Part model, mm, in its own coordinate system. A direction names the side the tool comes from. Coordinates: 2 decimals unless noted, no trailing zeros. Loops run counter-clockwise (first coordinate to the right, second up) from the corner with the lowest first, then second, coordinate; pieces in that order, holes last. Notation, with made-up numbers: (39.5, 80) -> (85.5, 80) arc R15 cw to (85.5, 98) -> close; hole circle Ø9 at (-0.75, -1.5). An arc over 180 degrees is marked (long way). One line per question, with ' | ' between items. Start each with the question number.
1) Cut at C-C (z = 51.5). List the corners of the cut face in (x, y), plus the area to 3 significant figures.
2) Cut at D-D (y = 26). Count the separate pieces of the cut face and the enclosed holes in it, plus the area to 3 significant figures.
3) Cut at A-A (x = 0). List the corners of the cut face in (y, z), plus the area to 4 significant figures.
4) Two-plate mould, pull along X, no slides. Class faces 1 (the face through (36.46, 0.8, 26.82)), 2 (the face through (31.457, -0.798, 58.2)), 3 (the face through (-65.41, 0.8, 3.84)), 4 (the face through (-1, 57, 99)): released by +X, released by -X, zero draft, split by the parting line, or undercut.
5) Drop flat-ended pins along their axis: pin 1 (4 mm diameter, centred on y = 22.5, z = 204, fed in from -X); pin 2 (11 mm diameter, centred on x = 65.5, y = 16.5, fed in from -Z); pin 3 (1 mm diameter, centred on y = -28.5, z = 88.5, fed in from +X). Give the stop position or say it passes through.
6) 3-axis set-ups, long thin cutter, end or side, ignore diameter. For faces 5 (the face through (-69, -1, 90)), 6 (the face through (-2.539, 19.334, 102.675)), 7 (the face through (31.86, 0.8, 223.22)), 8 (the face through (68, -1, 90)): which of +Z, -Z, +X, -X, +Y, -Y reach the whole face in a straight line?
7) Probe L1, parallel to Z at x = -17, y = -52; L2, parallel to Y at x = 0, z = 102; L3, parallel to Z at x = -6.5, y = -8. List the from-to ranges inside material, lowest first. Write a range as from..to.
from build123d import *

# Parameters (mm, degrees)
F1_DEPTH  = 57
F2_R      = 18
F3_R      = 10
F5_DEPTH  = 114
F6_R      = 5
F8_DEPTH  = 114
F9_R      = 10
F10_R     = 19.5
F11_DEPTH = 25


with BuildPart() as f1:
    # F0 (on Front) → F1 (new body, symmetric)
    with BuildSketch(Plane.XZ):
        Polygon((-70, 0), (70, 0), (50, 90), (112.991273, 90), (50, 250), (-50, 250), (-112.991273, 90), (-50, 90), align=None)
    extrude(amount=F1_DEPTH, both=True)

    # F2
    f2_edges = [f1.edges().sort_by_distance(p)[0] for p in [
        (50, 0, 250),
        (-50, 0, 250),
        (112.991273, 0, 90),
        (-112.991273, 0, 90),
    ]]
    fillet(f2_edges, radius=F2_R)

    # F3
    f3_edges = [f1.edges().sort_by_distance(p)[0] for p in [
        (70, 0, 0),
        (-70, 0, 0),
    ]]
    fillet(f3_edges, radius=F3_R)

    # F4 (on face) → F5 (cut, through all)
    with BuildSketch(Plane.XZ.offset(57)):
        Polygon((-38.834599, 25), (38.834599, 25), (24.390154, 90), (-24.390154, 90), align=None)
    extrude(amount=-F5_DEPTH, mode=Mode.SUBTRACT)

    # F6
    f6_edges = [f1.edges().sort_by_distance(p)[0] for p in [
        (-38.834599, 0, 25),
        (38.834599, 0, 25),
        (-24.390154, 0, 90),
        (24.390154, 0, 90),
    ]]
    fillet(f6_edges, radius=F6_R)

    # F7 (on face) → F8 (cut, through all)
    with BuildSketch(Plane.XZ.offset(57)):
        Polygon((-76.281201, 115), (76.281201, 115), (32.9747, 225), (-32.9747, 225), align=None)
    extrude(amount=-F8_DEPTH, mode=Mode.SUBTRACT)

    # F9
    f9_edges = [f1.edges().sort_by_distance(p)[0] for p in [
        (-76.281201, 0, 115),
        (76.281201, 0, 115),
        (32.9747, 0, 225),
        (-32.9747, 0, 225),
    ]]
    fillet(f9_edges, radius=F9_R)

    # F10 (on face) → F11 (cut, through all)
    with BuildSketch(Plane.XY.offset(115)):
        Circle(F10_R)
    extrude(amount=-F11_DEPTH, mode=Mode.SUBTRACT)


solid = f1.part
Reported:
1) outline: (-58.56, -57) -> (-32.95, -57) -> (-32.95, 57) -> (-58.56, 57) -> close; (32.95, -57) -> (58.56, -57) -> (58.56, 57) -> (32.95, 57) -> close | area: 5,840 mm²
2) separate pieces: 1 | enclosed holes: 2 | area: 20,400 mm²
3) outline: (-57, 0) -> (57, 0) -> (57, 25) -> (-57, 25) -> close; (-57, 90) -> (-19.5, 90) -> (-19.5, 115) -> (-57, 115) -> close; (-57, 225) -> (57, 225) -> (57, 250) -> (-57, 250) -> close; (19.5, 90) -> (57, 90) -> (57, 115) -> (19.5, 115) -> close | area: 7,575 mm²
4) face 1: undercut | face 2: undercut | face 3: released by -X | face 4: zero draft
5) pin 1: stops at x = -68.9 | pin 2: stops at z = 0.31 | pin 3: stops at x = 50.44
6) face 5: -X, +Y, -Y | face 6: none | face 7: +Y, -Y | face 8: +X, +Y, -Y
7) L1: z = 0..25, 90..115, 225..250 | L2: y = -57..-19.5, 19.5..57 | L3: z = 0..25, 225..250
